Design review of the part built by this model. Coordinates are the model's own, in mm. Face numbers are marked on the shaded views. A direction names the side the tool comes from. Coordinates: 2 decimals unless noted, no trailing zeros. Write each loop counter-clockwise with the first axis right and the second up, starting at its lowest first coordinate (ties: lowest second). Pieces come first, ordered by that corner, then holes.
Q1. Take a section at B-B, the plane x = 0. Write out the cut boundary in (y, z).
Q2. For L1, parallel to X at y = 1.05, z = -2; L2, parallel to X at y = 0.8, z = 1.25; L3, parallel to Y at x = -1.5, z = 1, list the stretches that pass through material, from the lowest coordinate up.
Q3. For pin 1 Ø1.5 at (y, z) = (2, -2) entering from -X; pin 2 Ø1 at (x, z) = (2, -1.5) entering from -Y, all flat-tipped, find the tip position at first contact; note any pin that passes through.
Q4. Take a section at A-A, the plane y = 0.95. Write out the cut boundary in (x, z).
Q5. Take a section at D-D, the plane x = 2.75. Write out the cut boundary in (y, z), plus the area to 3 significant figures.
Q6. The part is to be moulded in two halves that separate along X. For the marked faces 1, 2 and 3, say which applies: released by +X, released by -X, zero draft, split by the parting line, or undercut.
Q7. Take a section at C-C, the plane z = -2. Write out the cut boundary in (x, y).
Q8. For the marked faces 4, 5 and 6, list the 3-axis set-ups (+Z, -Z, +X, -X, +Y, -Y) from which the entire face can be reached by the end or side of a thin tool; tool diameter is ignored.
from build123d import *

# Parameters (mm, degrees)
ESQUISSE1_W           = 6.2
ESQUISSE1_H           = 6.4
BOSS_EXTRU_1_DEPTH    = 2
ESQUISSE2_R           = 1.65
BOSS_EXTRU_2_DEPTH    = 0.5
BOSS_EXTRU_4_START    = 1.3
BOSS_EXTRU_4_DEPTH    = 1.4
CONG_2_R              = 0.2
CONG_2_OF_SYM_TRIE2_R = 0.2
CONG_3_R              = 0.1
CONG_4_R              = 0.1


with BuildPart() as part:
    # Esquisse1 → Boss.-Extru.1 (new body)
    with BuildSketch(Plane(origin=(0, 0, 0), x_dir=(1, 0, 0), z_dir=(0, 1, 0))):
        Rectangle(ESQUISSE1_W, ESQUISSE1_H)
    extrude(amount=BOSS_EXTRU_1_DEPTH)

    # Esquisse2 → Boss.-Extru.2 (add)
    with BuildSketch(Plane(origin=(0, 2, 0), x_dir=(1, 0, 0), z_dir=(0, 1, 0))):
        with Locations(Location((0, 0, 0), (0, 0, 270))):
            Circle(ESQUISSE2_R)
    extrude(amount=BOSS_EXTRU_2_DEPTH)

    # Esquisse4 → Boss.-Extru.4 (add)
    with BuildSketch(Plane.XY.offset(BOSS_EXTRU_4_START)):
        Polygon((3.1, 0), (2.4, 0), (2.4, -0.1), (3.6, -0.1), (3.6, 1.1), (3.3, 1.1), (3.3, 0), align=None)
        Polygon((-2.4, -0.1), (-2.4, 0), (-3.3, 0), (-3.3, 1.1), (-3.6, 1.1), (-3.6, -0.1), align=None)
    boss_extru_4 = extrude(amount=BOSS_EXTRU_4_DEPTH)

    # Congé2
    # the kernel refuses this fillet: 0.2 mm, written as the material it takes off along each edge
    with BuildSketch(Plane(origin=(-2.4, -0.1, 0.866987298), x_dir=(0, 1, 0), z_dir=(0, 0, 1))) as cong_2_piece_1:
        with BuildLine():
            CenterArc((0.2, 0.173205081), CONG_2_R, 180, 60)
            Line((0, 0.173205081), (-0.004, 0.173205081))
            Line((-0.004, 0.173205081), (-0.004, 0))
            Line((-0.004, 0), (0, -0.004))
            ThreePointArc((0, -0.004), (0.05, -0.004), (0.098, -0.003464102))
            Line((0.098, -0.003464102), (0.1, 0))
        make_face()
    extrude(amount=2.266025404, mode=Mode.SUBTRACT)
    with BuildSketch(Plane(origin=(2.4, -0.1, 0.866987298), x_dir=(0, 1, 0), z_dir=(0, 0, 1))) as cong_2_piece_2:
        with BuildLine():
            CenterArc((0.2, -0.173205081), CONG_2_R, 120, 60)
            Line((0, -0.173205081), (-0.004, -0.173205081))
            Line((-0.004, -0.173205081), (-0.004, 0))
            Line((-0.004, 0), (0, 0.004))
            ThreePointArc((0, 0.004), (0.05, 0.004), (0.098, 0.003464102))
            Line((0.098, 0.003464102), (0.1, 0))
        make_face()
    extrude(amount=2.266025404, mode=Mode.SUBTRACT)
    with BuildSketch(Plane(origin=(3.6, -0.1, 0.8), x_dir=(0, 1, 0), z_dir=(0, 0, 1))) as cong_2_piece_3:
        with BuildLine():
            CenterArc((CONG_2_R, CONG_2_R), CONG_2_R, 180, 90)
            Line((0, CONG_2_R), (-CONG_2_R * 0.02, CONG_2_R))
            Line((-CONG_2_R * 0.02, CONG_2_R), (-CONG_2_R * 0.02, -CONG_2_R * 0.02))
            Line((-CONG_2_R * 0.02, -CONG_2_R * 0.02), (CONG_2_R, -CONG_2_R * 0.02))
            Line((CONG_2_R, -CONG_2_R * 0.02), (CONG_2_R, 0))
        make_face()
    extrude(amount=2.4, mode=Mode.SUBTRACT)
    with BuildSketch(Plane(origin=(-3.6, -0.1, 0.8), x_dir=(0, 1, 0), z_dir=(0, 0, 1))) as cong_2_piece_4:
        with BuildLine():
            CenterArc((CONG_2_R, -CONG_2_R), CONG_2_R, 90, 90)
            Line((0, -CONG_2_R), (-CONG_2_R * 0.02, -CONG_2_R))
            Line((-CONG_2_R * 0.02, -CONG_2_R), (-CONG_2_R * 0.02, CONG_2_R * 0.02))
            Line((-CONG_2_R * 0.02, CONG_2_R * 0.02), (CONG_2_R, CONG_2_R * 0.02))
            Line((CONG_2_R, CONG_2_R * 0.02), (CONG_2_R, 0))
        make_face()
    extrude(amount=2.4, mode=Mode.SUBTRACT)

    # Symétrie2: Boss.-Extru.4 across plane
    add(boss_extru_4.mirror(Plane.XY))

    # Congé2 of Symétrie2
    # the kernel refuses this fillet: 0.2 mm, written as the material it takes off along each edge
    with BuildSketch(Plane(origin=(-2.4, -0.1, -0.866987298), x_dir=(0, 1, 0), z_dir=(0, 0, -1))) as cong_2_of_sym_trie2_piece_1:
        with BuildLine():
            CenterArc((0.2, -0.173205081), CONG_2_OF_SYM_TRIE2_R, 120, 60)
            Line((0, -0.173205081), (-0.004, -0.173205081))
            Line((-0.004, -0.173205081), (-0.004, 0))
            Line((-0.004, 0), (0, 0.004))
            ThreePointArc((0, 0.004), (0.05, 0.004), (0.098, 0.003464102))
            Line((0.098, 0.003464102), (0.1, 0))
        make_face()
    extrude(amount=2.266025404, mode=Mode.SUBTRACT)
    with BuildSketch(Plane(origin=(2.4, -0.1, -0.866987298), x_dir=(0, 1, 0), z_dir=(0, 0, -1))) as cong_2_of_sym_trie2_piece_2:
        with BuildLine():
            CenterArc((0.2, 0.173205081), CONG_2_OF_SYM_TRIE2_R, 180, 60)
            Line((0, 0.173205081), (-0.004, 0.173205081))
            Line((-0.004, 0.173205081), (-0.004, 0))
            Line((-0.004, 0), (0, -0.004))
            ThreePointArc((0, -0.004), (0.05, -0.004), (0.098, -0.003464102))
            Line((0.098, -0.003464102), (0.1, 0))
        make_face()
    extrude(amount=2.266025404, mode=Mode.SUBTRACT)
    with BuildSketch(Plane(origin=(3.6, -0.1, -0.8), x_dir=(0, 1, 0), z_dir=(0, 0, -1))) as cong_2_of_sym_trie2_piece_3:
        with BuildLine():
            CenterArc((CONG_2_OF_SYM_TRIE2_R, -CONG_2_OF_SYM_TRIE2_R), CONG_2_OF_SYM_TRIE2_R, 90, 90)
            Line((0, -CONG_2_OF_SYM_TRIE2_R), (-CONG_2_OF_SYM_TRIE2_R * 0.02, -CONG_2_OF_SYM_TRIE2_R))
            Line((-CONG_2_OF_SYM_TRIE2_R * 0.02, -CONG_2_OF_SYM_TRIE2_R), (-CONG_2_OF_SYM_TRIE2_R * 0.02, CONG_2_OF_SYM_TRIE2_R * 0.02))
            Line((-CONG_2_OF_SYM_TRIE2_R * 0.02, CONG_2_OF_SYM_TRIE2_R * 0.02), (CONG_2_OF_SYM_TRIE2_R, CONG_2_OF_SYM_TRIE2_R * 0.02))
            Line((CONG_2_OF_SYM_TRIE2_R, CONG_2_OF_SYM_TRIE2_R * 0.02), (CONG_2_OF_SYM_TRIE2_R, 0))
        make_face()
    extrude(amount=2.4, mode=Mode.SUBTRACT)
    with BuildSketch(Plane(origin=(-3.6, -0.1, -0.8), x_dir=(0, 1, 0), z_dir=(0, 0, -1))) as cong_2_of_sym_trie2_piece_4:
        with BuildLine():
            CenterArc((CONG_2_OF_SYM_TRIE2_R, CONG_2_OF_SYM_TRIE2_R), CONG_2_OF_SYM_TRIE2_R, 180, 90)
            Line((0, CONG_2_OF_SYM_TRIE2_R), (-CONG_2_OF_SYM_TRIE2_R * 0.02, CONG_2_OF_SYM_TRIE2_R))
            Line((-CONG_2_OF_SYM_TRIE2_R * 0.02, CONG_2_OF_SYM_TRIE2_R), (-CONG_2_OF_SYM_TRIE2_R * 0.02, -CONG_2_OF_SYM_TRIE2_R * 0.02))
            Line((-CONG_2_OF_SYM_TRIE2_R * 0.02, -CONG_2_OF_SYM_TRIE2_R * 0.02), (CONG_2_OF_SYM_TRIE2_R, -CONG_2_OF_SYM_TRIE2_R * 0.02))
            Line((CONG_2_OF_SYM_TRIE2_R, -CONG_2_OF_SYM_TRIE2_R * 0.02), (CONG_2_OF_SYM_TRIE2_R, 0))
        make_face()
    extrude(amount=2.4, mode=Mode.SUBTRACT)

    # Congé3
    cong_3_edges = [part.edges().sort_by_distance(p)[0] for p in [
        (0, 2.5, -1.65),
    ]]
    fillet(cong_3_edges, radius=CONG_3_R)

    # Congé4
    cong_4_edges = [part.edges().sort_by_distance(p)[0] for p in [
        (3.1, 2, 0),
        (0, 2, -3.2),
        (-3.1, 2, 0),
        (0, 2, 3.2),
    ]]
    fillet(cong_4_edges, radius=CONG_4_R)


solid = part.part
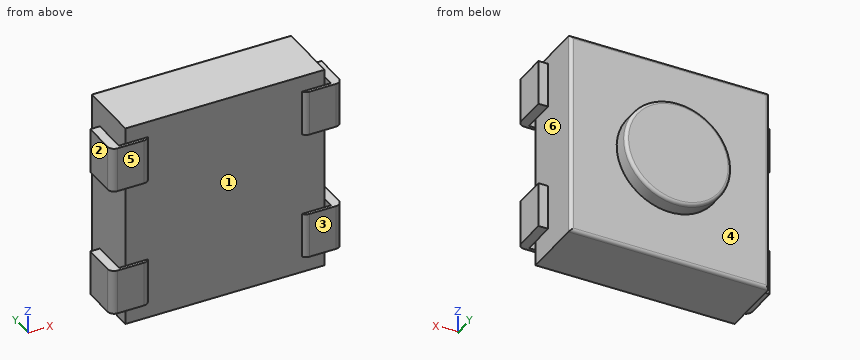
Responses:
1. outline: (0, -3.2) - (1.9, -3.2) arc R0.1 ccw to (2, -3.1) - (2, -1.65) - (2.4, -1.65) arc R0.1 ccw to (2.5, -1.55) - (2.5, 1.55) arc R0.1 ccw to (2.4, 1.65) - (2, 1.65) - (2, 3.1) arc R0.1 ccw to (1.9, 3.2) - (0, 3.2) - close
2. L1: x = -3.6 to -3.3, -3.1 to 3.1, 3.3 to 3.6
2. L2: x = -3.1 to 3.1
2. L3: y = 0 to 2
3. pin 1: stops at x = -3.1
3. pin 2: stops at y = -0.09
4. outline: (-3.6, -2.7) - (-3.3, -2.7) - (-3.3, -1.3) - (-3.6, -1.3) - close; (-3.6, 1.3) - (-3.3, 1.3) - (-3.3, 2.7) - (-3.6, 2.7) - close; (-3.1, -3.2) - (3.1, -3.2) - (3.1, 3.2) - (-3.1, 3.2) - close; (3.3, -2.7) - (3.6, -2.7) - (3.6, -1.3) - (3.3, -1.3) - close; (3.3, 1.3) - (3.6, 1.3) - (3.6, 2.7) - (3.3, 2.7) - close
5. outline: (-0.1, -2.7) - (0, -2.7) - (0, -3.2) - (1.9, -3.2) arc R0.1 ccw to (2, -3.1) - (2, 3.1) arc R0.1 ccw to (1.9, 3.2) - (0, 3.2) - (0, 2.7) - (-0.1, 2.7) - (-0.1, 1.3) - (0, 1.3) - (0, -1.3) - (-0.1, -1.3) - close
5. area: 13.1 mm2
6. face 1: undercut
6. face 2: released by -X
6. face 3: zero draft
7. outline: (-3.6, 0.1) arc R0.2 ccw to (-3.4, -0.1) - (-2.57, -0.1) arc R0.2 ccw to (-2.4, 0) - (2.4, 0) arc R0.2 ccw to (2.57, -0.1) - (3.4, -0.1) arc R0.2 ccw to (3.6, 0.1) - (3.6, 1.1) - (3.3, 1.1) - (3.3, 0) - (3.1, 0) - (3.1, 1.9) arc R0.1 ccw to (3, 2) - (-3, 2) arc R0.1 ccw to (-3.1, 1.9) - (-3.1, 0) - (-3.3, 0) - (-3.3, 1.1) - (-3.6, 1.1) - close
8. face 4: +Y
8. face 5: +Z, -Z, +X, -X, -Y
8. face 6: +Z, -Z, +Y
